Work out the finished part from the listing and answer in its coordinate system (mm). Coordinates: 2 decimals unless noted, no trailing zeros. Loops run counter-clockwise (first coordinate to the right, second up) from the corner with the lowest first, then second, coordinate; pieces in that order, holes last. Notation, with made-up numbers: (79.5, 56) -> (86.5, 56) arc R20 cw to (86.5, 90) -> close; hole circle Ø6 at (-39, -36). An arc over 180 degrees is marked (long way). Use a Markdown table: item, result. Add a question column.
```python
from build123d import *

# Parameters (mm, degrees)
SKETCH_1_R          = 52.5
SKETCH_1_R_2        = 2
SKETCH_1_R_3        = 2.5
EXTRUDE_1_DEPTH     = 3
CUT_EXTRUDE_1_DEPTH = 75.306796459
FILLET_1_R          = 5
FILLET_2_R          = 1
FILLET_3_R          = 2


with BuildPart() as part:
    # 草图1 → 凸台-拉伸1 (new body)
    with BuildSketch(Plane(origin=(0, 0, 0), x_dir=(1, 0, 0), z_dir=(0, 1, 0))):
        with Locations(Location((0, 0, 0), (0, 0, 270))):
            Circle(SKETCH_1_R)
        with Locations(Location((0, 49, 0), (0, 0, 270))):
            Circle(SKETCH_1_R_2, mode=Mode.SUBTRACT)
        with Locations(Location((-11.25, 19.485571585, 0), (0, 0, 270))):
            Circle(SKETCH_1_R_3, mode=Mode.SUBTRACT)
        with Locations(Location((42.435244785, 24.5, 0), (0, 0, 270))):
            Circle(SKETCH_1_R_2, mode=Mode.SUBTRACT)
        with Locations(Location((11.25, 19.485571585, 0), (0, 0, 270))):
            Circle(SKETCH_1_R_3, mode=Mode.SUBTRACT)
        with Locations(Location((42.435244785, -24.5, 0), (0, 0, 270))):
            Circle(SKETCH_1_R_2, mode=Mode.SUBTRACT)
        with Locations(Location((22.5, 0, 0), (0, 0, 270))):
            Circle(SKETCH_1_R_3, mode=Mode.SUBTRACT)
        with Locations(Location((0, -49, 0), (0, 0, 270))):
            Circle(SKETCH_1_R_2, mode=Mode.SUBTRACT)
        with Locations(Location((11.25, -19.485571585, 0), (0, 0, 270))):
            Circle(SKETCH_1_R_3, mode=Mode.SUBTRACT)
        with Locations(Location((-42.435244785, -24.5, 0), (0, 0, 270))):
            Circle(SKETCH_1_R_2, mode=Mode.SUBTRACT)
        with Locations(Location((-11.25, -19.485571585, 0), (0, 0, 270))):
            Circle(SKETCH_1_R_3, mode=Mode.SUBTRACT)
        with Locations(Location((-42.435244785, 24.5, 0), (0, 0, 270))):
            Circle(SKETCH_1_R_2, mode=Mode.SUBTRACT)
        with Locations(Location((-22.5, 0, 0), (0, 0, 270))):
            Circle(SKETCH_1_R_3, mode=Mode.SUBTRACT)
        with BuildLine():
            ThreePointArc((11.796996923, 12.925976311), (8.75, 15.155444566), (5.295725392, 16.679487179))
            ThreePointArc((5.295725392, 16.679487179), (4.40085173, 17.262951372), (3.933967434, 18.223809524))
            ThreePointArc((3.933967434, 18.223809524), (0, 21.5), (-3.933967434, 18.223809524))
            ThreePointArc((-3.933967434, 18.223809524), (-4.40085173, 17.262951372), (-5.295725392, 16.679487179))
            ThreePointArc((-5.295725392, 16.679487179), (-8.75, 15.155444566), (-11.796996923, 12.925976311))
            ThreePointArc((-11.796996923, 12.925976311), (-12.749728567, 12.442725082), (-13.815298284, 12.518820498))
            ThreePointArc((-13.815298284, 12.518820498), (-18.619546181, 10.75), (-17.749265718, 5.704989026))
            ThreePointArc((-17.749265718, 5.704989026), (-17.150580297, 4.820226289), (-17.092722316, 3.753510869))
            ThreePointArc((-17.092722316, 3.753510869), (-17.5, 0), (-17.092722316, -3.753510869))
            ThreePointArc((-17.092722316, -3.753510869), (-17.150580297, -4.820226289), (-17.749265718, -5.704989026))
            ThreePointArc((-17.749265718, -5.704989026), (-18.619546181, -10.75), (-13.815298284, -12.518820498))
            ThreePointArc((-13.815298284, -12.518820498), (-12.749728567, -12.442725082), (-11.796996923, -12.925976311))
            ThreePointArc((-11.796996923, -12.925976311), (-8.75, -15.155444566), (-5.295725392, -16.679487179))
            ThreePointArc((-5.295725392, -16.679487179), (-4.40085173, -17.262951372), (-3.933967434, -18.223809524))
            ThreePointArc((-3.933967434, -18.223809524), (0, -21.5), (3.933967434, -18.223809524))
            ThreePointArc((3.933967434, -18.223809524), (4.40085173, -17.262951372), (5.295725392, -16.679487179))
            ThreePointArc((5.295725392, -16.679487179), (8.75, -15.155444566), (11.796996923, -12.925976311))
            ThreePointArc((11.796996923, -12.925976311), (12.749728567, -12.442725082), (13.815298284, -12.518820498))
            ThreePointArc((13.815298284, -12.518820498), (18.619546181, -10.75), (17.749265718, -5.704989026))
            ThreePointArc((17.749265718, -5.704989026), (17.150580297, -4.820226289), (17.092722316, -3.753510869))
            ThreePointArc((17.092722316, -3.753510869), (17.5, 0), (17.092722316, 3.753510869))
            ThreePointArc((17.092722316, 3.753510869), (17.150580297, 4.820226289), (17.749265718, 5.704989026))
            ThreePointArc((17.749265718, 5.704989026), (18.619546181, 10.75), (13.815298284, 12.518820498))
            ThreePointArc((13.815298284, 12.518820498), (12.749728567, 12.442725082), (11.796996923, 12.925976311))
        make_face(mode=Mode.SUBTRACT)
    extrude(amount=EXTRUDE_1_DEPTH)

    # 草图2 → 切除-拉伸1 (cut, through all)
    with BuildSketch(Plane(origin=(0, 3, 0), x_dir=(1, 0, 0), z_dir=(0, 1, 0))):
        with BuildLine():
            Line((-6.071164737, 47.110412424), (-14.473042792, 25.068045456))
            Line((-14.473042792, 25.068045456), (-37.763231573, 28.812989105))
            ThreePointArc((-37.763231573, 28.812989105), (-23.75, 41.13620668), (-6.071164737, 47.110412424))
        make_face()
        with BuildLine():
            Line((0, 34.961858062), (3.494563236, 25.793854821))
            ThreePointArc((3.494563236, 25.793854821), (0, 26.5), (-3.494563236, 25.793854821))
            Line((-3.494563236, 25.793854821), (0, 34.961858062))
        make_face()
        with BuildLine():
            Line((14.473042792, 25.068045456), (6.071164737, 47.110412424))
            ThreePointArc((6.071164737, 47.110412424), (23.75, 41.13620668), (37.763231573, 28.812989105))
            Line((37.763231573, 28.812989105), (14.473042792, 25.068045456))
        make_face()
        with BuildLine():
            Line((30.277857245, 17.480929031), (20.590851919, 15.923307948))
            ThreePointArc((20.590851919, 15.923307948), (22.9496732, 13.25), (24.085415154, 9.870546873))
            Line((24.085415154, 9.870546873), (30.277857245, 17.480929031))
        make_face()
        with BuildLine():
            Line((28.946085584, 0), (43.83439631, 18.297423319))
            ThreePointArc((43.83439631, 18.297423319), (47.5, 0), (43.83439631, -18.297423319))
            Line((43.83439631, -18.297423319), (28.946085584, 0))
        make_face()
        with BuildLine():
            Line((30.277857245, -17.480929031), (24.085415154, -9.870546873))
            ThreePointArc((24.085415154, -9.870546873), (22.9496732, -13.25), (20.590851919, -15.923307948))
            Line((20.590851919, -15.923307948), (30.277857245, -17.480929031))
        make_face()
        with BuildLine():
            Line((14.473042792, -25.068045456), (37.763231573, -28.812989105))
            ThreePointArc((37.763231573, -28.812989105), (23.75, -41.13620668), (6.071164737, -47.110412424))
            Line((6.071164737, -47.110412424), (14.473042792, -25.068045456))
        make_face()
        with BuildLine():
            Line((0, -34.961858062), (3.494563236, -25.793854821))
            ThreePointArc((3.494563236, -25.793854821), (0, -26.5), (-3.494563236, -25.793854821))
            Line((-3.494563236, -25.793854821), (0, -34.961858062))
        make_face()
        with BuildLine():
            Line((-14.473042792, -25.068045456), (-6.071164737, -47.110412424))
            ThreePointArc((-6.071164737, -47.110412424), (-23.75, -41.13620668), (-37.763231573, -28.812989105))
            Line((-37.763231573, -28.812989105), (-14.473042792, -25.068045456))
        make_face()
        with BuildLine():
            Line((-30.277857245, -17.480929031), (-20.590851919, -15.923307948))
            ThreePointArc((-20.590851919, -15.923307948), (-22.9496732, -13.25), (-24.085415154, -9.870546873))
            Line((-24.085415154, -9.870546873), (-30.277857245, -17.480929031))
        make_face()
        with BuildLine():
            Line((-28.946085584, 0), (-43.83439631, -18.297423319))
            ThreePointArc((-43.83439631, -18.297423319), (-47.5, 0), (-43.83439631, 18.297423319))
            Line((-43.83439631, 18.297423319), (-28.946085584, 0))
        make_face()
        with BuildLine():
            Line((-30.277857245, 17.480929031), (-24.085415154, 9.870546873))
            ThreePointArc((-24.085415154, 9.870546873), (-22.9496732, 13.25), (-20.590851919, 15.923307948))
            Line((-20.590851919, 15.923307948), (-30.277857245, 17.480929031))
        make_face()
    extrude(amount=-CUT_EXTRUDE_1_DEPTH, mode=Mode.SUBTRACT)

    # 圆角1
    fillet_1_edges = [part.edges().sort_by_distance(p)[0] for p in [
        (-14.473042792, 1.5, 25.068045456),
        (14.473042792, 1.5, 25.068045456),
        (28.946085584, 1.5, 0),
        (14.473042792, 1.5, -25.068045456),
        (-28.946085584, 1.5, 0),
        (-14.473042792, 1.5, -25.068045456),
    ]]
    fillet(fillet_1_edges, radius=FILLET_1_R)

    # 圆角2
    fillet_2_edges = [part.edges().sort_by_distance(p)[0] for p in [
        (0, 1.5, 34.961858062),
        (-3.494563236, 1.5, 25.793854821),
        (3.494563236, 1.5, 25.793854821),
        (30.277857245, 1.5, 17.480929031),
        (20.590851919, 1.5, 15.923307948),
        (24.085415154, 1.5, 9.870546873),
        (30.277857245, 1.5, -17.480929031),
        (24.085415154, 1.5, -9.870546873),
        (20.590851919, 1.5, -15.923307948),
        (-3.494563236, 1.5, -25.793854821),
        (0, 1.5, -34.961858062),
        (3.494563236, 1.5, -25.793854821),
        (-30.277857245, 1.5, -17.480929031),
        (-20.590851919, 1.5, -15.923307948),
        (-24.085415154, 1.5, -9.870546873),
        (-30.277857245, 1.5, 17.480929031),
        (-24.085415154, 1.5, 9.870546873),
        (-20.590851919, 1.5, 15.923307948),
    ]]
    fillet(fillet_2_edges, radius=FILLET_2_R)

    # 圆角3
    fillet_3_edges = [part.edges().sort_by_distance(p)[0] for p in [
        (-6.071164737, 1.5, 47.110412424),
        (-37.763231573, 1.5, 28.812989105),
        (37.763231573, 1.5, 28.812989105),
        (6.071164737, 1.5, 47.110412424),
        (43.83439631, 1.5, -18.297423319),
        (43.83439631, 1.5, 18.297423319),
        (6.071164737, 1.5, -47.110412424),
        (37.763231573, 1.5, -28.812989105),
        (-43.83439631, 1.5, 18.297423319),
        (-43.83439631, 1.5, -18.297423319),
        (-37.763231573, 1.5, -28.812989105),
        (-6.071164737, 1.5, -47.110412424),
    ]]
    fillet(fillet_3_edges, radius=FILLET_3_R)


solid = part.part
```
Item 1: Given pin 1 (3 mm diameter, centred on x = -22.5, z = 0, fed in from -Y), flat-ended and moving along its own axis, determine where the tip first touches the part or whether it passes through.
Item 2: For a pull along X with two mould halves and no side action, classify faces 1 (the face through (-26.97, 1.521, 13.415)), 2 (the face through (-23.57, 1.52, 41.24)), 3 (the face through (1, 3, 23)) as +X half, -X half, draft (parallel to the pull), parting line (faces both ways), or undercut.
Item 3: Section A-A (z = -24) is taken. Determine the outline of the cut face in (x, y), then the cut area to 3 significant figures.
Item 4: Find the intervals of material crossed by probe 1 along X at (y, z) = (2.3, -21); probe 2 along Z at (x, y) = (-28, 1.6); probe 3 along Z at (x, y) = (35.5, 2.4), in increasing order.
Item 5: Section C-C (y = 0.75) is taken. Count the separate pieces of the cut face and the enclosed holes in it, then the cut area to 3 significant figures.
Item 6: Section B-B (z = 49) is taken. Determine the outline of the cut face in (x, y), then the cut area to 3 significant figures.
Output:
| question | item | result |
|---|---|---|
| 1 | pin 1 | passes through |
| 2 | face 1 | undercut |
| 2 | face 2 | undercut |
| 2 | face 3 | draft |
| 3 | outline | (-46.69, 0) -> (-44.37, 0) -> (-44.37, 3) -> (-46.69, 3) -> close; (-40.5, 0) -> (40.5, 0) -> (40.5, 3) -> (-40.5, 3) -> close; (44.37, 0) -> (46.69, 0) -> (46.69, 3) -> (44.37, 3) -> close |
| 3 | area | 257 mm2 |
| 4 | probe 1 | x = -48.12 to -13.24, -9.26 to -1.94, 1.94 to 9.26, 13.24 to 48.12 |
| 4 | probe 2 | z = -44.41 to -38.37, -27.24 to -17.07, -14.68 to 14.68, 17.07 to 27.24, 38.37 to 44.41 |
| 4 | probe 3 | z = -38.68 to -31.56, -28.91 to -8.05, 8.05 to 28.91, 31.56 to 38.68 |
| 5 | separate pieces | 1 |
| 5 | enclosed holes | 25 |
| 5 | area | 5,070 mm2 |
| 6 | outline | (-18.85, 0) -> (-2, 0) -> (-2, 3) -> (-18.85, 3) -> close; (2, 0) -> (18.85, 0) -> (18.85, 3) -> (2, 3) -> close |
| 6 | area | 101 mm2 |
